Design review of the part built by this model. Coordinates are the model's own, in mm. Round coordinates to 2 decimals unless told otherwise and drop trailing zeros. Loops run counter-clockwise (first coordinate to the right, second up) from the corner with the lowest first, then second, coordinate; pieces in that order, holes last. Notation, with made-up numbers: (33.25, -21) - (91.25, -21) arc R27 cw to (91.25, 9) - close; hole circle Ø5 at (0, 16). An arc over 180 degrees is marked (long way). Return JSON: item names as keys, results as strings. Group by question number.
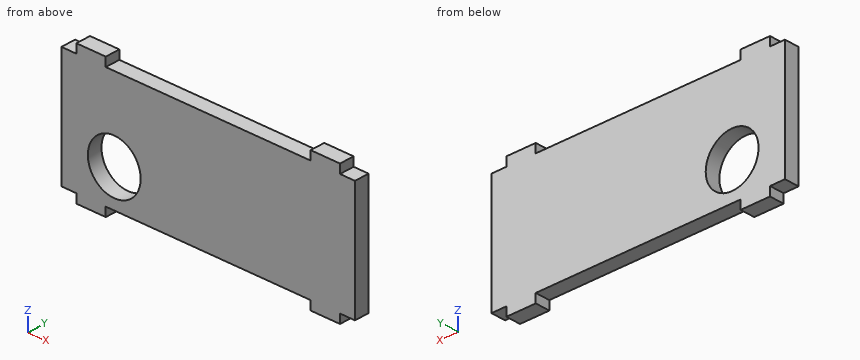
Autodesk Inventor part; units mm, degrees
ref_plane "YZ Plane" through (0, 0, 0) normal (1, 0, 0) x (0, 1, 0)
ref_plane "XZ Plane" through (0, 0, 0) normal (0, 1, 0) x (-1, 0, 0)
ref_plane "XY Plane" through (0, 0, 0) normal (0, 0, 1) x (1, 0, 0)
sketch "Sketch1" plane through (0, 0, 0) normal (0, 1, 0) x (-1, 0, 0)
  line L0 (0, 0) -> (100, 0)
  line L1 (100, 0) -> (100, -40)
  line L2 (100, -40) -> (0, -40)
  line L3 (0, -40) -> (0, 0)
  line L4 (94.9, -40) -> (84.9, -40)
  line L5 (84.9, -40) -> (84.9, -43)
  line L6 (84.9, -43) -> (94.9, -43)
  line L7 (94.9, -43) -> (94.9, -40)
  line L8 (15.1, -40) -> (5.1, -40)
  line L9 (5.1, -40) -> (5.1, -43)
  line L10 (5.1, -43) -> (15.1, -43)
  line L11 (15.1, -43) -> (15.1, -40)
  line L12 (15.1, 0) -> (5.1, 0)
  line L13 (5.1, 0) -> (5.1, 3)
  line L14 (5.1, 3) -> (15.1, 3)
  line L15 (15.1, 3) -> (15.1, 0)
  line L16 (84.9, 0) -> (94.9, 0)
  line L17 (94.9, 0) -> (94.9, 3)
  line L18 (94.9, 3) -> (84.9, 3)
  line L19 (84.9, 3) -> (84.9, 0)
  dimension "d0" = 40
  dimension "d1" = 100
  dimension "d2" = 3
  dimension "d3" = 5.1
  dimension "d4" = 10
  dimension "d5" = 5.1
  dimension "d6" = 10
  dimension "d7" = 5.1
  dimension "d8" = 3
  dimension "d9" = 5.1
  dimension "d10" = 10
extrude "Extrusion1" add sketch "Sketch1" along normal blind 5
sketch "Sketch2" plane through (0, 0, 0) normal (0, -1, 0) x (1, 0, 0)
  circle A0 centre (-82, -27.5) radius 9
  line L0 (-100, -40) -> (-100, 0)
  line L1 (-15.1, -40) -> (-84.9, -40)
  point P0 (0, 0)
  dimension "d13" = 18
  dimension "d14" = 18
  dimension "d15" = 12.5
extrude "Extrusion2" cut sketch "Sketch2" against normal blind 5
properties part number "Steckerplatte_seit"
Q1. Add section C-C, the plane x = -82. State the section outline as (y, z) points.
Q2. Add section A-A, the plane y = 4.05. State the section outline as (x, z) points.
Q3. For line 1 (X direction, y = 3.55, z = -27); line 2 (Z direction, x = -82, y = 2.85); line 3 (X direction, y = 3.05, z = -30.5), list the stretches that pass through material, from the lowest coordinate up.
Q4. Add section B-B, the plane z = -27.5. State the section outline as (x, y) points.
Q5. Add section D-D, the plane x = -64. State the section outline as (y, z) points, plus the area to 3 significant figures.
Q6. Insertion check: pin 1 Ø2 at (x, y) = (-65, 0.5) entering from -Z; pin 2 Ø0.9 at (y, z) = (1.5, 1) entering from +X; pin 3 Ø2.5 at (x, y) = (-2.5, 2) entering from +Z. Each pin has a flat end and moves straight along its axis. Give the tip position at first contact, or say it passes through.
Evaluation:
{
 "1": {"outline": "(0, -40) - (5, -40) - (5, -36.5) - (0, -36.5) - close; (0, -18.5) - (5, -18.5) - (5, 0) - (0, 0) - close"},
 "2": {"outline": "(-100, -40) - (-94.9, -40) - (-94.9, -43) - (-84.9, -43) - (-84.9, -40) - (-15.1, -40) - (-15.1, -43) - (-5.1, -43) - (-5.1, -40) - (0, -40) - (0, 0) - (-5.1, 0) - (-5.1, 3) - (-15.1, 3) - (-15.1, 0) - (-84.9, 0) - (-84.9, 3) - (-94.9, 3) - (-94.9, 0) - (-100, 0) - close; hole circle Ø18 at (-82, -27.5)"},
 "3": {"line 1": "-100 to -90.99, -73.01 to 0", "line 2": "-40 to -36.5, -18.5 to 0", "line 3": "-100 to -90.49, -73.51 to 0"},
 "4": {"outline": "(-100, 0) - (-91, 0) - (-91, 5) - (-100, 5) - close; (-73, 0) - (0, 0) - (0, 5) - (-73, 5) - close"},
 "5": {"outline": "(0, -40) - (5, -40) - (5, 0) - (0, 0) - close", "area": "200 mm²"},
 "6": {"pin 1": "z = -40", "pin 2": "x = -5.1", "pin 3": "z = 0"}
}
